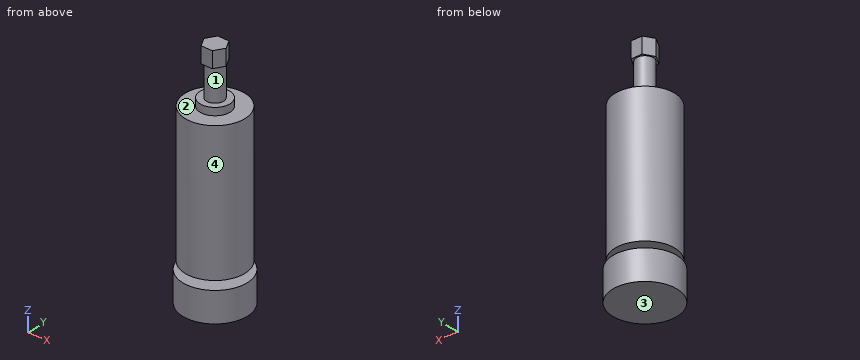
```python
from build123d import *

# Parameters (mm, degrees)
ESQUISSE1_R        = 26
BOSS_EXTRU_1_DEPTH = 120
ESQUISSE2_R        = 13
BOSS_EXTRU_2_DEPTH = 6.5
BOSS_EXTRU_3_START = 6.5
ESQUISSE3_R        = 13
BOSS_EXTRU_3_DEPTH = 6.5
ESQUISSE4_R        = 7.5
BOSS_EXTRU_4_DEPTH = 28
BOSS_EXTRU_5_DEPTH = 14
ESQUISSE6_R        = 28
BOSS_EXTRU_6_DEPTH = 26


with BuildPart() as part:
    # Esquisse1 → Boss.-Extru.1 (new body)
    with BuildSketch(Plane.XY):
        Circle(ESQUISSE1_R)
    extrude(amount=BOSS_EXTRU_1_DEPTH)

    # Esquisse2 → Boss.-Extru.2 (add)
    with BuildSketch(Plane.XY.offset(120)):
        with Locations(Location((0, 0, 0), (0, 0, 180))):
            Circle(ESQUISSE2_R)
    extrude(amount=BOSS_EXTRU_2_DEPTH)

    # Esquisse3 → Boss.-Extru.3 (add)
    with BuildSketch(Plane(origin=(0, 0, 0), x_dir=(-1, 0, 0), z_dir=(0, 0, -1)).offset(BOSS_EXTRU_3_START)):
        Circle(ESQUISSE3_R)
    extrude(amount=-BOSS_EXTRU_3_DEPTH)

    # Esquisse4 → Boss.-Extru.4 (add)
    with BuildSketch(Plane.XY.offset(126.5)):
        Circle(ESQUISSE4_R)
    extrude(amount=BOSS_EXTRU_4_DEPTH)

    # Esquisse5 → Boss.-Extru.5 (add)
    with BuildSketch(Plane.XY.offset(154.5)):
        Polygon((9.814954576, 0), (4.907477288, 8.5), (-4.907477288, 8.5), (-9.814954576, 0), (-4.907477288, -8.5), (4.907477288, -8.5), align=None)
    extrude(amount=BOSS_EXTRU_5_DEPTH)

    # Esquisse6 → Boss.-Extru.6 (add)
    with BuildSketch(Plane(origin=(0, 0, -6.5), x_dir=(-1, 0, 0), z_dir=(0, 0, -1))):
        Circle(ESQUISSE6_R)
    extrude(amount=BOSS_EXTRU_6_DEPTH)


solid = part.part
```
Geometry: final body of the model. Coordinates: model frame, mm. Face numbers are marked on the shaded views. Round coordinates to 2 decimals unless told otherwise and drop trailing zeros. Loops run counter-clockwise (first coordinate to the right, second up) from the corner with the lowest first, then second, coordinate; pieces in that order, holes last. Notation, with made-up numbers: (-8, 84.5) -> (4, 84.5) arc R13 ccw to (4, 90.5) -> close; hole circle Ø3 at (-7, 20). An arc over 180 degrees is marked (long way). Write each question's results on one line, items separated by ' | '.
Item 1: Cut plane B-B on x = -17.5. Return the cut outline in (y, z).
Answers below:
outline: (-21.86, -32.5) -> (21.86, -32.5) -> (21.86, -6.5) -> (-21.86, -6.5) -> close; (-19.23, 0) -> (19.23, 0) -> (19.23, 120) -> (-19.23, 120) -> close
Item 2: Pull-direction query (Z, two-part tool) for the marked faces 1, 2, 3 and 4; classes: pulls with the +Z half, pulls with the -Z half, needs draft (parallel to the pull), parting line crosses it, or undercut.
Answers below:
face 1: undercut | face 2: pulls with the +Z half | face 3: pulls with the -Z half | face 4: needs draft
Item 3: Pin query (flat end, axial travel): pin 1 Ø5 at (x, z) = (-2, 161) entering from +Y; pin 2 Ø2 at (x, y) = (-19.5, -11) entering from +Z; pin 3 Ø4 at (x, y) = (1.5, 13) entering from +Z. Return the tip coordinate at first contact, or that it passes through.
Answers below:
pin 1: stops at y = 8.5 | pin 2: stops at z = 120 | pin 3: stops at z = 126.5
Item 4: Cut plane A-A on x = 0. Return the cut outline in (y, z).
Answers below:
outline: (-28, -32.5) -> (28, -32.5) -> (28, -6.5) -> (13, -6.5) -> (13, 0) -> (26, 0) -> (26, 120) -> (13, 120) -> (13, 126.5) -> (7.5, 126.5) -> (7.5, 154.5) -> (8.5, 154.5) -> (8.5, 168.5) -> (-8.5, 168.5) -> (-8.5, 154.5) -> (-7.5, 154.5) -> (-7.5, 126.5) -> (-13, 126.5) -> (-13, 120) -> (-26, 120) -> (-26, 0) -> (-13, 0) -> (-13, -6.5) -> (-28, -6.5) -> close
Item 5: Line query: probe 1 along Z at (x, y) = (2, -22); probe 2 along Z at (x, y) = (12.5, -24.5); probe 3 along Y at (x, z) = (-0.5, 33). Output: solid intervals per line, ascending. Write a range as [from, to].
Answers below:
probe 1: z = [-32.5, -6.5], [0, 120] | probe 2: z = [-32.5, -6.5] | probe 3: y = [-26, 26]
Item 6: Cut plane D-D on y = -3.5. Return the cut outline in (x, z).
Answers below:
outline: (-27.78, -32.5) -> (27.78, -32.5) -> (27.78, -6.5) -> (12.52, -6.5) -> (12.52, 0) -> (25.76, 0) -> (25.76, 120) -> (12.52, 120) -> (12.52, 126.5) -> (6.63, 126.5) -> (6.63, 154.5) -> (7.79, 154.5) -> (7.79, 168.5) -> (-7.79, 168.5) -> (-7.79, 154.5) -> (-6.63, 154.5) -> (-6.63, 126.5) -> (-12.52, 126.5) -> (-12.52, 120) -> (-25.76, 120) -> (-25.76, 0) -> (-12.52, 0) -> (-12.52, -6.5) -> (-27.78, -6.5) -> close
Item 7: Cut plane C-C on y = 20.5. Return the cut outline in (x, z).
Answers below:
outline: (-19.07, -32.5) -> (19.07, -32.5) -> (19.07, -6.5) -> (-19.07, -6.5) -> close; (-15.99, 0) -> (15.99, 0) -> (15.99, 120) -> (-15.99, 120) -> close
